Design review of the part built by this model. Coordinates are the model's own, in mm. A direction names the side the tool comes from. Coordinates: 2 decimals unless noted, no trailing zeros. Loops run counter-clockwise (first coordinate to the right, second up) from the corner with the lowest first, then second, coordinate; pieces in that order, holes last. Notation, with made-up numbers: (-7, -26) - (10, -26) arc R5 ccw to (10, -18) - close; hole circle Ø11 at (-11.75, 59.5). An arc over 180 degrees is marked (long way). Answer in a Markdown table with one row per item. Add a question column.
(1) Clearance check with flat-ended pins moving along their axes: pin 1 (1.5 mm diameter, centred on x = -1.5, y = -1.5, fed in from +Z); pin 2 (1.5 mm diameter, centred on x = -0.5, z = 2.5, fed in from +Y). State where each tip first meets the part, or that it passes through.
(2) We need section A-A, the plane z = 3.75. Write out the cut boundary in (x, y).
(3) To check wall thickness, follow L1, parallel to Z at x = -1.3, y = 2.05; L2, parallel to Y at x = -0.1, z = 3; L3, parallel to Z at x = 1.45, y = -1.7. State the ranges of each line that lie inside material, in increasing order. Write a range as [from, to].
(4) For faces 1 (the face through (-0.54, -2.44, 0.38)), 2 (the face through (-1.825, -1.4, 2.901)), list the 3-axis set-ups (+Z, -Z, +X, -X, +Y, -Y) from which the entire face can be reached by the end or side of a thin tool; tool diameter is ignored.
from build123d import *

# Parameters (mm, degrees)
SKETCH_R     = 2.5
PAD_DEPTH    = 0.762
SKETCH002_R  = 2.3
PAD001_DEPTH = 5.1


with BuildPart() as part:
    # Sketch → Pad (new body)
    with BuildSketch(Plane.XY):
        Circle(SKETCH_R)
    extrude(amount=PAD_DEPTH)

    # Sketch002 → Pad001 (join)
    with BuildSketch(Plane.XY):
        Circle(SKETCH002_R)
    extrude(amount=PAD001_DEPTH)

    # Sketch003 → Revolution (revolve)
    with BuildSketch(Plane.YZ):
        with BuildLine():
            Line((0, 5.1), (0, 6.4))
            ThreePointArc((2.133073, 5.1), (1.249, 6.04939), (0, 6.4))
            Line((0, 5.1), (2.133073, 5.1))
        make_face()
    revolve(axis=Axis((0, 0, 0), (0, 0, 1)))


solid = part.part
Responses:
| question | item | result |
|---|---|---|
| 1 | pin 1 | stops at z = 5.97 |
| 1 | pin 2 | stops at y = 2.3 |
| 2 | outline | circle Ø4.6 at (0, 0) |
| 3 | L1 | z = [0, 0.76] |
| 3 | L2 | y = [-2.3, 2.3] |
| 3 | L3 | z = [0, 5.1] |
| 4 | face 1 | +Z, -Z |
| 4 | face 2 | +Z |
